For this review, take the finished solid that the model builds, in its own axes (mm). A direction names the side the tool comes from. Give positions to 0.01 mm unless a question says otherwise; leave off trailing zeros. Loops run counter-clockwise (first coordinate to the right, second up) from the corner with the lowest first, then second, coordinate; pieces in that order, holes last. Notation, with made-up numbers: (-17, 50.25) - (-8, 50.25) arc R33 cw to (-8, 88.25) - close; hole circle Ø10 at (-13, 71.25). An arc over 180 degrees is marked (long way). Put each result on its own line as item: value.
from build123d import *

# Parameters (mm, degrees)
F0_R       = 31.75
F1_DEPTH   = 393.7
F3_R       = 19.05
F4_DEPTH   = 35.052
F1_FACE_R  = 31.75
F4_FACE_R  = 19.05
F1_FACE1_R = 31.75
F5_FACE_R  = 19.05
F9_D       = 12.7
F9_DEPTH   = 44.45
F9_TIP     = 3.8154649308
F11_D      = 12.7
F11_DEPTH  = 44.45
F11_TIP    = 3.8154649308


with BuildPart() as f1:
    # F0 (on Right) → F1 (new body, symmetric)
    with BuildSketch(Plane.YZ):
        Circle(F0_R)
    extrude(amount=F1_DEPTH, both=True)



with BuildPart() as f4:
    # F3 (on offset) → F4 (new body)
    with BuildSketch(Plane.YZ.offset(536.448)):
        Circle(F3_R)
    extrude(amount=-F4_DEPTH)


with BuildPart() as f5_1:
    # F5: instance of F4
    add(f4.part.mirror(Plane.YZ))


with BuildPart() as f1_1:
    add(f1.part)

    add(f4.part)  # F6 merges F4
    # F1_face (on face) → F6 section 0
    with BuildSketch(Plane.YZ.offset(393.7)):
        Circle(F1_FACE_R)
    # F4_face (on face) → F6 section 1
    with BuildSketch(Plane(origin=(501.396, 0, 0), x_dir=(0, 1, 0), z_dir=(-1, 0, 0))):
        Circle(F4_FACE_R)
    loft()


    add(f5_1.part)  # F7 merges F5_1
    # F1_face1 (on face) → F7 section 0
    with BuildSketch(Plane(origin=(-393.7, 0, 0), x_dir=(0, 1, 0), z_dir=(-1, 0, 0))):
        Circle(F1_FACE1_R)
    # F5_face (on face) → F7 section 1
    with BuildSketch(Plane.YZ.offset(-501.396)):
        Circle(F5_FACE_R)
    loft()

    # F9
    with Locations(Plane.YZ.offset(536.448)):
        with Locations((0, 0)):
            Hole(F9_D / 2, depth=F9_DEPTH)
            with Locations((0, 0, -(F9_DEPTH + F9_TIP / 2))):  # 118° drill point
                Cone(0, F9_D / 2, F9_TIP, mode=Mode.SUBTRACT)

    # F11
    with Locations(Plane(origin=(-536.448, 0, 0), x_dir=(0, -1, 0), z_dir=(-1, 0, 0))):
        with Locations((0, 0)):
            Hole(F11_D / 2, depth=F11_DEPTH)
            with Locations((0, 0, -(F11_DEPTH + F11_TIP / 2))):  # 118° drill point
                Cone(0, F11_D / 2, F11_TIP, mode=Mode.SUBTRACT)


solid = f1_1.part
1) For faces 1 (the face through (519.17, -15.12, -11.59)), 2 (the face through (-536.448, -5, 5)), 3 (the face through (-519.17, -15.12, -11.59)), list the 3-axis set-ups (+Z, -Z, +X, -X, +Y, -Y) from which the entire face can be reached by the end or side of a thin tool; tool diameter is ignored.
Geometry check:
face 1: +X
face 2: +Z, -Z, -X, +Y, -Y
face 3: -X
2) Wall thickness on line 1 (Z direction, x = 503, y = 0); line 2 (Z direction, x = 59, y = 0.5); line 3 (Z direction, x = 486.5, y = -10): over which ranges is each line inside the solid? List them lowest first.
Geometry check:
line 1: z = -19.05 to -6.35, 6.35 to 19.05
line 2: z = -31.75 to 31.75
line 3: z = -18.25 to 18.25
3) Take a section at A-A on x = -246. State the section outline as (y, z) points, and give its area (3 significant figures).
Geometry check:
outline: circle Ø63.5 at (0, 0)
area: 3,170 mm²
4) Insertion check: pin 1 Ø3 at (x, y) = (-324.5, 6.5) entering from +Z; pin 2 Ø11.5 at (y, z) = (0, 0) entering from +X; pin 3 Ø2 at (x, z) = (-29.5, 8.5) entering from +Y. Each pin has a flat end and moves straight along its axis. Give the tip position at first contact, or say it passes through.
Geometry check:
pin 1: stops at z = 31.35
pin 2: stops at x = 491.64
pin 3: stops at y = 30.85
